```python
from build123d import *

# Parameters (mm, degrees)
BOSS_EXTRUDE1_DEPTH = 160
BOSS_EXTRUDE2_START = -12
SKETCH2_W           = 60
SKETCH2_H           = 72
BOSS_EXTRUDE2_DEPTH = 76
FILLET1_RADIUS      = 30
FILLET1_LENGTH      = 76
SKETCH3_R           = 15
CUT_EXTRUDE1_DEPTH  = 76
RIB1_REACH          = 190.404
SKETCH4_WALL_W      = 512.089299886
SKETCH4_WALL_H      = 12


with BuildPart() as part:
    # Sketch1 → Boss-Extrude1 (new body)
    with BuildSketch(Plane.XY):
        Polygon((26, 0), (-26, 0), (-26, -10), (-50, -10), (-50, 0), (-38, 0), (-38, 14), (38, 14), (38, 2), (50, 2), (50, -10), (26, -10), align=None)
    extrude(amount=BOSS_EXTRUDE1_DEPTH)

    # Sketch2 → Boss-Extrude2 (add)
    with BuildSketch(Plane(origin=(50, 0, 0), x_dir=(0, 0, -1), z_dir=(1, 0, 0)).offset(BOSS_EXTRUDE2_START)):
        with Locations((-30, 50)):
            Rectangle(SKETCH2_W, SKETCH2_H)
    extrude(amount=-BOSS_EXTRUDE2_DEPTH)

    # Fillet1: full round fillet: the end face becomes a half cylinder, R = half its width
    fillet1_face = Plane((0, 86, 30), x_dir=(1, 0, 0), z_dir=(0, 1, 0))  # on the end face: x along it, z out of the body
    fillet1_slab = fillet1_face.offset(-FILLET1_RADIUS / 2) * Box(FILLET1_LENGTH, 2 * FILLET1_RADIUS, FILLET1_RADIUS, mode=Mode.PRIVATE)  # the body's end, R deep
    fillet1_round = Plane((0, 56, 30), x_dir=(0, 1, 0), z_dir=(1, 0, 0)) * Cylinder(FILLET1_RADIUS, FILLET1_LENGTH, mode=Mode.PRIVATE)  # its axis R under the face
    add(fillet1_slab - fillet1_round, mode=Mode.SUBTRACT)

    # Sketch3 → Cut-Extrude1 (cut)
    with BuildSketch(Plane(origin=(38, 0, 0), x_dir=(0, 0, -1), z_dir=(1, 0, 0))):
        with Locations((-30, 56)):
            Circle(SKETCH3_R)
    extrude(amount=-CUT_EXTRUDE1_DEPTH, mode=Mode.SUBTRACT)

    # Sketch4 wall → Rib1 (add, up to next)
    with BuildSketch(Plane(origin=(0, 47.912517706, 102.633274951), x_dir=(0, -0.508884996756, 0.860834513758), z_dir=(0, -0.860834513758, -0.508884996756)), mode=Mode.PRIVATE) as rib1_sk1:
        Rectangle(SKETCH4_WALL_W, SKETCH4_WALL_H)
    rib1_tool1 = extrude(rib1_sk1.sketch, amount=RIB1_REACH, mode=Mode.PRIVATE) - part.part
    add(rib1_tool1.solids().sort_by_distance((0, 47.912517706, 102.633274951))[0])


solid = part.part
```
Geometry check sheet. Reference: the model listing, model coordinates, mm. A direction names the side the tool comes from. Coordinates: 2 decimals unless noted, no trailing zeros. Write each loop counter-clockwise with the first axis right and the second up, starting at its lowest first coordinate (ties: lowest second). Pieces come first, ordered by that corner, then holes. Notation, with made-up numbers: M 70,-17 L 85,-17 A24 ccw 85,0 Z; hole C 81.5,6 d11. An arc over 180 degrees is marked long. One line per item, written item: value. Start each with the question number.
(1) Depth check by flat-ended pin: pin 1 (3.5 mm diameter, centred on x = 41.5, z = 107, fed in from +Y); pin 2 (6 mm diameter, centred on x = -43, z = 52.5, fed in from +Y); pin 3 (12 mm diameter, centred on x = -30, z = 131.5, fed in from +Y). Enter the tip coordinate at first touch or a pass-through.
(2) Tool access check on faces 4 (the face through (-6, 32, 92)), 5 (the face through (-38, 30, 51)), 6 (the face through (0.532, 85.993, 29.34)). Record the directions out of +Z, -Z, +X, -X, +Y, -Y that give a thin tool (end or side, any length) a straight path to the whole face; none if there is none.
(3) Sectioned sample at D-D, the plane x = -1.5. Enter the section's corners in (y, z).
(4) Release check for a two-part mould opening along X. For faces 1 (the face through (1, 5, 160)), 2 (the face through (38, 29, 51)), 3 (the face through (26, -5, 79)) record: released by +X, released by -X, zero draft, split by the parting line, or undercut.
(5) Sectioned sample at B-B, the plane x = -18.5. Enter the section's corners in (y, z), and give its area (3 significant figures).
(6) Sectioned sample at C-C, the plane y = 36.5. Enter the section's corners in (x, z), and give its area (3 significant figures).
(7) Sectioned sample at A-A, the plane z = 30. Enter the section's corners in (x, y).
(8) Scan lines: line 1 along Y through (x, z) = (11, 30); line 2 along X through (y, z) = (38, 9.5); line 3 along Y through (x, z) = (-35, 101). Record each from-to range of solid material in increasing order. Write a range as [from, to].
Filled sheet:
1. pin 1: y = 2
1. pin 2: y = 0
1. pin 3: y = 14
2. face 4: +Z, -X, +Y
2. face 5: +Z, -Z, -X, +Y
2. face 6: +Y
3. outline: M 0,0 L 56,0 A30 ccw 81.83,45.27 L 14,160 L 0,160 Z; hole C 56,30 d30
4. face 1: zero draft
4. face 2: released by +X
4. face 3: undercut
5. outline: M 0,0 L 56,0 A30 ccw 56,60 L 14,60 L 14,160 L 0,160 Z; hole C 56,30 d30
5. area: 5,470 mm²
6. outline: M -38,0 L 38,0 L 38,60 L 6,60 L 6,121.94 L -6,121.94 L -6,60 L -38,60 Z
6. area: 5,300 mm²
7. outline: M -50,-10 L -26,-10 L -26,0 L 26,0 L 26,-10 L 50,-10 L 50,2 L 38,2 L 38,41 L -38,41 L -38,0 L -50,0 Z; M -38,71 L 38,71 L 38,86 L -38,86 Z
8. line 1: [0, 41], [71, 86]
8. line 2: [-38, 38]
8. line 3: [-10, 14]
